from build123d import *

# Parameters (mm, degrees)
BOSS_EXTRUDE1_DEPTH      = 20
SHELL1_T                 = -10
SHELL1_THICKNESS_2_DEPTH = 6
SKETCH3_R                = 32.5
CUT_EXTRUDE5_DEPTH       = 119.84864324
CUT_EXTRUDE6_DEPTH       = 119.84864324
SKETCH5_R                = 17.5
CUT_EXTRUDE7_DEPTH       = 119.84864324
SKETCH6_R                = 1.7
BOSS_EXTRUDE2_DEPTH      = 50
SKETCH6_2_R              = 1.7
CUT_EXTRUDE8_DEPTH       = 35
SKETCH9_R                = 1.7
BOSS_EXTRUDE3_DEPTH      = 32.5
SKETCH9_2_R              = 1.7
CUT_EXTRUDE10_DEPTH      = 12.75
CUT_EXTRUDE9_DEPTH       = 2
FILLET1_R                = 5
FILLET2_R                = 0.5
SKETCH10_W               = 46.141745146
SKETCH10_H               = 188.45260123
CUT_EXTRUDE11_DEPTH      = 186.270073136


with BuildPart() as part:
    # Sketch1 → Boss-Extrude1 (new body)
    with BuildSketch(Plane.XY):
        with BuildLine():
            Line((55, -90), (-55, -90))
            ThreePointArc((-55, -90), (-69.142135624, -84.142135624), (-75, -70))
            Line((-75, -70), (-75, 70))
            ThreePointArc((-75, 70), (-69.142135624, 84.142135624), (-55, 90))
            Line((-55, 90), (55, 90))
            ThreePointArc((55, 90), (69.142135624, 84.142135624), (75, 70))
            Line((75, 70), (75, -70))
            ThreePointArc((75, -70), (69.142135624, -84.142135624), (55, -90))
        make_face()
    extrude(amount=BOSS_EXTRUDE1_DEPTH)

    # Shell1
    shell1_openings = [part.faces().sort_by_distance(p)[0] for p in [
        (0, 0, 20),
    ]]
    offset(amount=SHELL1_T, openings=shell1_openings, kind=Kind.INTERSECTION)

    # Shell1 thickness 2 face (on inner face of the shell) → Shell1 thickness 2 (cut)
    with BuildSketch(Plane(origin=(0, 0, 10), x_dir=(-1, 0, 0), z_dir=(0, 0, -1))):
        with BuildLine():
            ThreePointArc((-55, -80), (-62.071067812, -77.071067812), (-65, -70))
            Line((-65, -70), (-65, 70))
            ThreePointArc((-65, 70), (-62.071067812, 77.071067812), (-55, 80))
            Line((-55, 80), (55, 80))
            ThreePointArc((55, 80), (62.071067812, 77.071067812), (65, 70))
            Line((65, 70), (65, -70))
            ThreePointArc((65, -70), (62.071067812, -77.071067812), (55, -80))
            Line((55, -80), (-55, -80))
        make_face()
    extrude(amount=SHELL1_THICKNESS_2_DEPTH, mode=Mode.SUBTRACT)

    # Sketch3 → Cut-Extrude5 (cut, through all)
    with BuildSketch(Plane.XY):
        with Locations(Location((0, -36.75, 0), (0, 0, 180))):
            Circle(SKETCH3_R)
    extrude(amount=CUT_EXTRUDE5_DEPTH, mode=Mode.SUBTRACT)

    # Sketch4 → Cut-Extrude6 (cut, through all)
    with BuildSketch(Plane.XY):
        with BuildLine():
            Line((-30.75, 13.25), (-9.25, 13.25))
            ThreePointArc((-9.25, 13.25), (-8.542893219, 13.542893219), (-8.25, 14.25))
            Line((-8.25, 14.25), (-8.25, 35.75))
            ThreePointArc((-8.25, 35.75), (-8.542893219, 36.457106781), (-9.25, 36.75))
            Line((-9.25, 36.75), (-30.75, 36.75))
            ThreePointArc((-30.75, 36.75), (-31.457106781, 36.457106781), (-31.75, 35.75))
            Line((-31.75, 35.75), (-31.75, 14.25))
            ThreePointArc((-31.75, 14.25), (-31.457106781, 13.542893219), (-30.75, 13.25))
        make_face()
    extrude(amount=CUT_EXTRUDE6_DEPTH, mode=Mode.SUBTRACT)

    # Sketch5 → Cut-Extrude7 (cut, through all)
    with BuildSketch(Plane.XY):
        with Locations(Location((20, 25, 0), (0, 0, 180))):
            Circle(SKETCH5_R)
    extrude(amount=CUT_EXTRUDE7_DEPTH, mode=Mode.SUBTRACT)

    # Sketch6 → Boss-Extrude2 (add, symmetric)
    with BuildSketch(Plane(origin=(0, 0, 0), x_dir=(1, 0, 0), z_dir=(0, 1, 0))):
        with BuildLine():
            Line((75, -20), (75, -10))
            ThreePointArc((75, -10), (76.464466094, -13.535533906), (80, -15))
            ThreePointArc((80, -15), (83.535533906, -23.535533906), (75, -20))
        make_face()
        with Locations(Location((80, -20, 0), (0, 0, 270))):
            Circle(SKETCH6_R, mode=Mode.SUBTRACT)
    extrude(amount=BOSS_EXTRUDE2_DEPTH, both=True)

    # Sketch6_2 → Cut-Extrude8 (cut, symmetric)
    with BuildSketch(Plane(origin=(0, 0, 0), x_dir=(1, 0, 0), z_dir=(0, 1, 0))):
        with BuildLine():
            Line((75, -20), (75, -10))
            ThreePointArc((75, -10), (76.464466094, -13.535533906), (80, -15))
            ThreePointArc((80, -15), (83.535533906, -23.535533906), (75, -20))
        make_face()
        with Locations(Location((80, -20, 0), (0, 0, 270))):
            Circle(SKETCH6_2_R, mode=Mode.SUBTRACT)
    extrude(amount=CUT_EXTRUDE8_DEPTH, both=True, mode=Mode.SUBTRACT)

    # Sketch9 → Boss-Extrude3 (add, symmetric)
    with BuildSketch(Plane(origin=(0, 0, 0), x_dir=(1, 0, 0), z_dir=(0, 1, 0))):
        with BuildLine():
            Line((-75, -10), (-75, -20))
            ThreePointArc((-75, -20), (-83.535533906, -23.535533906), (-80, -15))
            ThreePointArc((-80, -15), (-76.464466094, -13.535533906), (-75, -10))
        make_face()
        with Locations(Location((-80, -20, 0), (0, 0, 270))):
            Circle(SKETCH9_R, mode=Mode.SUBTRACT)
    extrude(amount=BOSS_EXTRUDE3_DEPTH, both=True)

    # Sketch9_2 → Cut-Extrude10 (cut, symmetric)
    with BuildSketch(Plane(origin=(0, 0, 0), x_dir=(1, 0, 0), z_dir=(0, 1, 0))):
        with BuildLine():
            Line((-75, -10), (-75, -20))
            ThreePointArc((-75, -20), (-83.535533906, -23.535533906), (-80, -15))
            ThreePointArc((-80, -15), (-76.464466094, -13.535533906), (-75, -10))
        make_face()
        with Locations(Location((-80, -20, 0), (0, 0, 270))):
            Circle(SKETCH9_2_R, mode=Mode.SUBTRACT)
    extrude(amount=CUT_EXTRUDE10_DEPTH, both=True, mode=Mode.SUBTRACT)

    # Sketch7 → Cut-Extrude9 (cut)
    with BuildSketch(Plane.XY.offset(4)):
        with BuildLine():
            Line((-26, -0.75), (26, -0.75))
            ThreePointArc((26, -0.75), (33.071067812, -3.678932188), (36, -10.75))
            Line((36, -10.75), (36, -62.75))
            ThreePointArc((36, -62.75), (33.071067812, -69.821067812), (26, -72.75))
            Line((26, -72.75), (-26, -72.75))
            ThreePointArc((-26, -72.75), (-33.071067812, -69.821067812), (-36, -62.75))
            Line((-36, -62.75), (-36, -10.75))
            ThreePointArc((-36, -10.75), (-33.071067812, -3.678932188), (-26, -0.75))
        make_face()
        with BuildLine():
            Line((8, 47), (32, 47))
            ThreePointArc((32, 47), (39.071067812, 44.071067812), (42, 37))
            Line((42, 37), (42, 13))
            ThreePointArc((42, 13), (39.071067812, 5.928932188), (32, 3))
            Line((32, 3), (8, 3))
            ThreePointArc((8, 3), (0.928932188, 5.928932188), (-2, 13))
            Line((-2, 13), (-2, 37))
            ThreePointArc((-2, 37), (0.928932188, 44.071067812), (8, 47))
        make_face()
    extrude(amount=-CUT_EXTRUDE9_DEPTH, mode=Mode.SUBTRACT)

    # Fillet1
    fillet1_edges = [part.edges().sort_by_distance(p)[0] for p in [
        (0, -90, 0),
        (-69.142135624, -84.142135624, 0),
        (-62.071067812, -77.071067812, 4),
        (0, -80, 4),
        (62.071067812, -77.071067812, 4),
        (65, 0, 4),
        (62.071067812, 77.071067812, 4),
        (0, 80, 4),
        (-62.071067812, 77.071067812, 4),
        (-65, 0, 4),
        (-75, 0, 0),
        (-69.142135624, 84.142135624, 0),
        (0, 90, 0),
        (69.142135624, 84.142135624, 0),
        (75, 0, 0),
        (69.142135624, -84.142135624, 0),
    ]]
    fillet(fillet1_edges, radius=FILLET1_R)

    # Fillet2
    fillet2_edges = [part.edges().sort_by_distance(p)[0] for p in [
        (69.142135624, -84.142135624, 20),
        (75, 0, 20),
        (-75, -51.25, 20),
        (75, -60, 20),
        (-75, 0, 20),
        (-33.071067812, -69.821067812, 4),
        (0, -72.75, 4),
        (33.071067812, -69.821067812, 4),
        (36, -36.75, 4),
        (33.071067812, -3.678932188, 4),
        (0, -0.75, 4),
        (-33.071067812, -3.678932188, 4),
        (-36, -36.75, 4),
        (69.142135624, 84.142135624, 20),
        (0.928932188, 5.928932188, 4),
        (20, 3, 4),
        (39.071067812, 5.928932188, 4),
        (42, 25, 4),
        (39.071067812, 44.071067812, 4),
        (20, 47, 4),
        (0.928932188, 44.071067812, 4),
        (-2, 25, 4),
        (0, 90, 20),
        (-69.142135624, 84.142135624, 20),
        (-75, 51.25, 20),
        (-62.071067812, -77.071067812, 20),
        (0, -80, 20),
        (62.071067812, -77.071067812, 20),
        (65, 0, 20),
        (62.071067812, 77.071067812, 20),
        (0, 80, 20),
        (-62.071067812, 77.071067812, 20),
        (-65, 0, 20),
        (-69.142135624, -84.142135624, 20),
        (32.5, -36.75, 0),
        (-8.542893219, 13.542893219, 0),
        (-8.25, 25, 0),
        (-8.542893219, 36.457106781, 0),
        (-20, 36.75, 0),
        (-31.457106781, 36.457106781, 0),
        (-31.75, 25, 0),
        (-31.457106781, 13.542893219, 0),
        (-20, 13.25, 0),
        (0, -90, 20),
        (37.5, 25, 0),
        (75, 60, 20),
    ]]
    fillet(fillet2_edges, radius=FILLET2_R)

    # Sketch10 → Cut-Extrude11 (cut, through all)
    with BuildSketch(Plane.ZY.offset(75)):
        with Locations((9.585784517, 0.121425645)):
            Rectangle(SKETCH10_W, SKETCH10_H)
    extrude(amount=-CUT_EXTRUDE11_DEPTH, mode=Mode.SUBTRACT)


with BuildPart() as body_2:
    # of the pieces the cut leaves, the one that is kept (cut_extrude11_keep)
    add(part.part.solids().sort_by_distance((-75, 12.75, 20))[0])


solid = body_2.part
Geometry: final body of the model. Coordinates: model frame, mm. Give positions to 0.01 mm unless a question says otherwise; leave off trailing zeros. Order: outer loops, then holes, each group sorted by start corner. A loop starts at its lowest first (then second) coordinate and runs counter-clockwise, first axis right, second up. Notation, with made-up numbers: (46, 82.25) -> (75, 82.25) arc R22 ccw to (75, 92.25) -> close; hole circle Ø6 at (-27.75, 38). An arc over 180 degrees is marked (long way). Write each question's results on one line, items separated by ' | '.
1) Cut plane A-A (z = 20.5). Output: boundary loops of the cut face in (x, y), and give its area (3 significant figures).
Geometry says:
outline: (-84.97, 12.75) -> (-81.62, 12.75) -> (-81.62, 32.5) -> (-84.97, 32.5) -> close; (-78.38, 12.75) -> (-75.03, 12.75) -> (-75.03, 32.5) -> (-78.38, 32.5) -> close | area: 132 mm²
2) Line query: line 1 along X through (y, z) = (24.5, 20); line 2 along Z through (x, y) = (-80, 25.5); line 3 along X through (y, z) = (30.5, 18.5). Output: solid intervals per line, ascending.
Geometry says:
line 1: x = -85 to -81.7, -78.3 to -75 | line 2: z = 15 to 18.3, 21.7 to 25 | line 3: x = -84.77 to -80.8, -79.2 to -75
3) Cut plane C-C (x = -76.25). Output: boundary loops of the cut face in (y, z).
Geometry says:
outline: (12.75, 13.31) -> (32.5, 13.31) -> (32.5, 23.31) -> (12.75, 23.31) -> close
4) First-contact query: pin 1 Ø4 at (x, y) = (-81.5, 16.5) entering from -Z; pin 2 Ø1 at (x, z) = (-77.5, 13.5) entering from +Y; pin 3 Ø4 at (x, y) = (-81, 26) entering from -Z; pin 4 Ø3 at (y, z) = (24, 22) entering from -X. Flat tips, straight axial feed; report the tip coordinate or a pass-through.
Geometry says:
pin 1: stops at z = 14.97 | pin 2: passes through | pin 3: stops at z = 14.9 | pin 4: stops at x = -84.97
5) Cut plane D-D (z = 16.5). Output: boundary loops of the cut face in (x, y).
Geometry says:
outline: (-83.57, 12.75) -> (-75, 12.75) -> (-75, 32.5) -> (-83.57, 32.5) -> close
6) Cut plane B-B (y = 28.5). Output: boundary loops of the cut face in (x, z).
Geometry says:
outline: (-80, 15) arc R5 cw to (-75, 10) -> (-75, 20) arc R5 ccw (long way) to start; hole circle Ø3.4 at (-80, 20)
7) Draft query along X for faces 1 (the face through (-75, 23, 15)), 2 (the face through (-78, 12.75, 19)), 3 (the face through (-81.5, 22.5, 20.8)). Return one class per face: released by +X, released by -X, zero draft, split by the parting line, or undercut.
Geometry says:
face 1: released by +X | face 2: zero draft | face 3: undercut
